Geometry check sheet. Reference: the model listing, model coordinates, mm. Face numbers are marked on the shaded views. Give positions to 0.01 mm unless a question says otherwise; leave off trailing zeros. Loops run counter-clockwise (first coordinate to the right, second up) from the corner with the lowest first, then second, coordinate; pieces in that order, holes last. Notation, with made-up numbers: (16.5, 28.25) - (47.5, 28.25) arc R22 ccw to (47.5, 62.25) - close; hole circle Ø1 at (-29.75, 28.25). An arc over 180 degrees is marked (long way). Use a Markdown table: item, result. Add a question column.
1. Cross-section at A-A on x = 1321.75. Enter the section's corners in (y, z).
2. Draft check along X on the marked faces 1 and 2. Enter one of: pulls with the +X half, pulls with the -X half, needs draft (parallel to the pull), parting line crosses it, or undercut.
3. Depth check by flat-ended pin: P1, Ø2, axis at y = 1018, z = 86.5, coming from the +X side; P2, Ø5.5, axis at y = 1014, z = 62.5, coming from the +X side; P3, Ø5.5, axis at y = 1014.5, z = 99, coming from the +X side. Enter the tip coordinate at first touch or a pass-through.
4. Cross-section at B-B on z = 10. Enter the section's corners in (x, y), and give its area (3 significant figures).
5. Material ranges on L1, parallel to Y at x = 1326.5, z = 52.5; L2, parallel to Y at x = 1319.6, z = 46; L3, parallel to X at y = 1008, z = 33.5, recorded low to high.
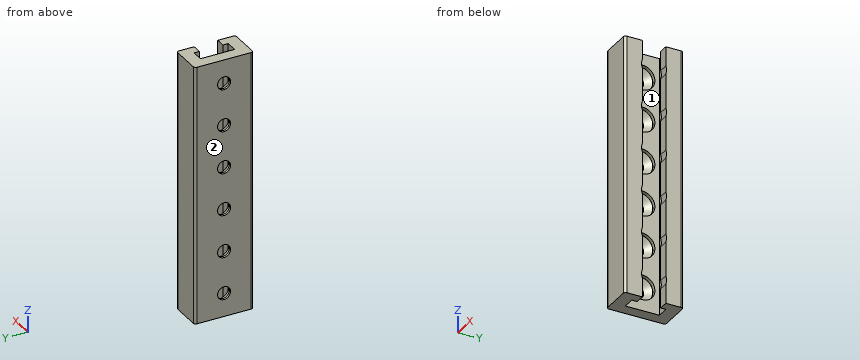
from build123d import *

# Parameters (mm, degrees)
EXTRUDE_1_DEPTH     = 110
SKETCH_2_R          = 2.75
CUT_EXTRUDE_2_DEPTH = 110
SKETCH_3_R          = 5.3
CUT_EXTRUDE_3_DEPTH = 10.6
CHAMFER_1_SIZE      = 2.5
CHAMFER_2_SIZE      = 2.5
CHAMFER_3_SIZE      = 2.5
CHAMFER_4_SIZE      = 2.5
CHAMFER_5_SIZE      = 2.5
CHAMFER_6_SIZE      = 2.5


with BuildPart() as part:
    # 草图1 → 拉伸1 (new body)
    with BuildSketch(Plane.XY):
        with BuildLine():
            Line((1315.337068447, 1002.71396169), (1315.337068447, 1025.71396169))
            ThreePointArc((1315.337068447, 1025.71396169), (1315.629961666, 1026.421068471), (1316.337068447, 1026.71396169))
            Line((1316.337068447, 1026.71396169), (1328.337068447, 1026.71396169))
            ThreePointArc((1328.337068447, 1026.71396169), (1329.044175228, 1026.421068471), (1329.337068447, 1025.71396169))
            Line((1329.337068447, 1025.71396169), (1329.337068447, 1019.21396169))
            Line((1329.337068447, 1019.21396169), (1325.337068447, 1019.21396169))
            Line((1325.337068447, 1019.21396169), (1325.337068447, 1021.46396169))
            Line((1325.337068447, 1021.46396169), (1320.337068447, 1021.46396169))
            Line((1320.337068447, 1021.46396169), (1320.337068447, 1006.96396169))
            Line((1320.337068447, 1006.96396169), (1325.337068447, 1006.96396169))
            Line((1325.337068447, 1006.96396169), (1325.337068447, 1009.21396169))
            Line((1325.337068447, 1009.21396169), (1329.337068447, 1009.21396169))
            Line((1329.337068447, 1009.21396169), (1329.337068447, 1002.71396169))
            ThreePointArc((1329.337068447, 1002.71396169), (1329.044175228, 1002.006854909), (1328.337068447, 1001.71396169))
            Line((1328.337068447, 1001.71396169), (1316.337068447, 1001.71396169))
            ThreePointArc((1316.337068447, 1001.71396169), (1315.629961666, 1002.006854909), (1315.337068447, 1002.71396169))
        make_face()
    extrude(amount=EXTRUDE_1_DEPTH)

    # 草图2 → 拉伸2 (cut)
    with BuildSketch(Plane.ZY.offset(-1315.337068447)):
        with Locations((100, 1014.21396169)):
            Circle(SKETCH_2_R)
        with Locations((82, 1014.21396169)):
            Circle(SKETCH_2_R)
        with Locations((64, 1014.21396169)):
            Circle(SKETCH_2_R)
        with Locations((46, 1014.21396169)):
            Circle(SKETCH_2_R)
        with Locations((28, 1014.21396169)):
            Circle(SKETCH_2_R)
        with Locations((10, 1014.21396169)):
            Circle(SKETCH_2_R)
    extrude(amount=-CUT_EXTRUDE_2_DEPTH, mode=Mode.SUBTRACT)

    # 草图3 → 拉伸3 (cut)
    with BuildSketch(Plane(origin=(1329.337068447, 0, 0), x_dir=(0, 0, -1), z_dir=(1, 0, 0))):
        with Locations((-100, 1014.21396169)):
            Circle(SKETCH_3_R)
        with Locations((-82, 1014.21396169)):
            Circle(SKETCH_3_R)
        with Locations((-64, 1014.21396169)):
            Circle(SKETCH_3_R)
        with Locations((-46, 1014.21396169)):
            Circle(SKETCH_3_R)
        with Locations((-28, 1014.21396169)):
            Circle(SKETCH_3_R)
        with Locations((-10, 1014.21396169)):
            Circle(SKETCH_3_R)
    extrude(amount=-CUT_EXTRUDE_3_DEPTH, mode=Mode.SUBTRACT)

    # 倒角1
    chamfer_1_edges = [part.edges().sort_by_distance(p)[0] for p in [
        (1318.737068447, 1014.21396169, 97.25),
    ]]
    chamfer(chamfer_1_edges, length=CHAMFER_1_SIZE)

    # 倒角2
    chamfer_2_edges = [part.edges().sort_by_distance(p)[0] for p in [
        (1318.737068447, 1014.21396169, 79.25),
    ]]
    chamfer(chamfer_2_edges, length=CHAMFER_2_SIZE)

    # 倒角3
    chamfer_3_edges = [part.edges().sort_by_distance(p)[0] for p in [
        (1318.737068447, 1014.21396169, 61.25),
    ]]
    chamfer(chamfer_3_edges, length=CHAMFER_3_SIZE)

    # 倒角4
    chamfer_4_edges = [part.edges().sort_by_distance(p)[0] for p in [
        (1318.737068447, 1014.21396169, 43.25),
    ]]
    chamfer(chamfer_4_edges, length=CHAMFER_4_SIZE)

    # 倒角5
    chamfer_5_edges = [part.edges().sort_by_distance(p)[0] for p in [
        (1318.737068447, 1014.21396169, 25.25),
    ]]
    chamfer(chamfer_5_edges, length=CHAMFER_5_SIZE)

    # 倒角6
    chamfer_6_edges = [part.edges().sort_by_distance(p)[0] for p in [
        (1318.737068447, 1014.21396169, 7.25),
    ]]
    chamfer(chamfer_6_edges, length=CHAMFER_6_SIZE)


solid = part.part
Values found:
| question | item | result |
|---|---|---|
| 1 | outline | (1001.71, 0) - (1006.96, 0) - (1006.96, 110) - (1001.71, 110) - close; (1021.46, 0) - (1026.71, 0) - (1026.71, 110) - (1021.46, 110) - close |
| 2 | face 1 | undercut |
| 2 | face 2 | pulls with the -X half |
| 3 | P1 | stops at x = 1320.34 |
| 3 | P2 | stops at x = 1317.75 |
| 3 | P3 | stops at x = 1317.28 |
| 4 | outline | (1315.34, 1002.71) arc R1 ccw to (1316.34, 1001.71) - (1328.34, 1001.71) arc R1 ccw to (1329.34, 1002.71) - (1329.34, 1008.91) - (1325.34, 1008.91) - (1325.34, 1006.96) - (1320.34, 1006.96) - (1320.34, 1008.91) - (1318.74, 1008.91) - (1318.74, 1008.96) - (1316.24, 1011.46) - (1315.34, 1011.46) - close; (1315.34, 1016.96) - (1316.24, 1016.96) - (1318.74, 1019.46) - (1318.74, 1019.51) - (1320.34, 1019.51) - (1320.34, 1021.46) - (1325.34, 1021.46) - (1325.34, 1019.51) - (1329.34, 1019.51) - (1329.34, 1025.71) arc R1 ccw to (1328.34, 1026.71) - (1316.34, 1026.71) arc R1 ccw to (1315.34, 1025.71) - close |
| 4 | area | 192 mm2 |
| 5 | L1 | y = 1001.71 to 1009.21, 1019.21 to 1026.71 |
| 5 | L2 | y = 1001.71 to 1008.91, 1019.51 to 1026.71 |
| 5 | L3 | x = 1315.34 to 1320.34, 1325.34 to 1329.34 |
